For this review, take the finished solid that the model builds, in its own axes (mm). Face numbers are marked on the shaded views. A direction names the side the tool comes from. Give positions to 0.01 mm unless a question says otherwise; leave off trailing zeros. Write each loop counter-clockwise with the first axis right and the second up, starting at its lowest first coordinate (ties: lowest second). Pieces come first, ordered by that corner, then holes.
Q1. Mouldability with a two-part tool opening along Z and no side actions: class the marked faces 1, 2 and 3 as released by +Z, released by -Z, zero draft, split by the parting line, or undercut.
Q2. We need section A-A (x = 0). Write out the cut boundary in (y, z), then the cut area to 3 significant figures.
Q3. Machinability: for the marked faces 4 and 5, which of the approach directions +Z, -Z, +X, -X, +Y, -Y give a long, thin tool a straight path to every point of the face, cutting with its end or side? Answer none if there is none.
Q4. We need section B-B (z = 0). Write out the cut boundary in (x, y).
Q5. For line 1 (Y direction, x = 0.6, z = -0.15); line 2 (Y direction, x = 1.8, z = 0.45); line 3 (Z direction, x = -0.05, y = 1), list the stretches that pass through material, from the lowest coordinate up.
Q6. Insertion check: P1, Ø1, axis at x = -1, y = 8.5, coming from the +Z side; P2, Ø1, axis at y = 9, z = 1, coming from the +X side; P3, Ø1.5, axis at y = 3.5, z = 1, coming from the -X side. Each pin has a flat end and moves straight along its axis. Give the tip position at first contact, or say it passes through.
Q7. We need section C-C (y = 3). Write out the cut boundary in (x, z), then the cut area to 3 significant figures.
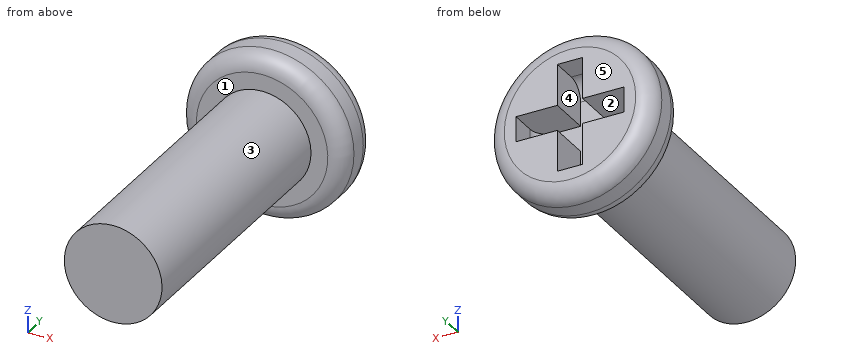
```python
from build123d import *

# Parameters (mm, degrees)
SKETCH1_R           = 1.45
BOSS_EXTRUDE1_DEPTH = 8
SKETCH2_R           = 2.45
BOSS_EXTRUDE2_DEPTH = 1.5
FILLET1_R           = 0.5
SKETCH3_W           = 0.75
SKETCH3_H           = 1.225
SKETCH3_H_2         = 0.75
SKETCH3_W_2         = 1.225
CUT_EXTRUDE1_DEPTH  = 1.25
FILLET4_R           = 0.5


with BuildPart() as part:
    # Sketch1 → Boss-Extrude1 (new body)
    with BuildSketch(Plane(origin=(0, 0, 0), x_dir=(1, 0, 0), z_dir=(0, 1, 0))):
        with Locations(Location((0, 0, 0), (0, 0, 270))):
            Circle(SKETCH1_R)
    extrude(amount=BOSS_EXTRUDE1_DEPTH)

    # Sketch2 → Boss-Extrude2 (add)
    with BuildSketch(Plane(origin=(0, 8, 0), x_dir=(1, 0, 0), z_dir=(0, 1, 0))):
        with Locations(Location((0, 0, 0), (0, 0, 270))):
            Circle(SKETCH2_R)
    extrude(amount=BOSS_EXTRUDE2_DEPTH)

    # Fillet1
    fillet1_edges = [part.edges().sort_by_distance(p)[0] for p in [
        (0, 8, -2.45),
        (0, 9.5, -2.45),
    ]]
    fillet(fillet1_edges, radius=FILLET1_R)

    # Sketch3 → Cut-Extrude1 (cut)
    with BuildSketch(Plane(origin=(0, 9.5, 0), x_dir=(1, 0, 0), z_dir=(0, 1, 0))):
        with Locations((0, 0.9875)):
            Rectangle(SKETCH3_W, SKETCH3_H)
        Rectangle(SKETCH3_W, SKETCH3_H_2)
        with Locations((0, -0.9875)):
            Rectangle(SKETCH3_W, SKETCH3_H)
        with Locations((0.9875, 0)):
            Rectangle(SKETCH3_W_2, SKETCH3_H_2)
        with Locations((-0.9875, 0)):
            Rectangle(SKETCH3_W_2, SKETCH3_H_2)
    extrude(amount=-CUT_EXTRUDE1_DEPTH, mode=Mode.SUBTRACT)

    # Fillet4
    fillet4_edges = [part.edges().sort_by_distance(p)[0] for p in [
        (0, 8.25, 1.6),
        (-1.6, 8.25, 0),
        (0, 8.25, -1.6),
        (1.6, 8.25, 0),
    ]]
    fillet(fillet4_edges, radius=FILLET4_R)


solid = part.part
```
Computed:
1. face 1: zero draft
1. face 2: undercut
1. face 3: split by the parting line
2. outline: (0, -1.45) - (8, -1.45) - (8, -1.95) arc R0.5 ccw to (8.5, -2.45) - (9, -2.45) arc R0.5 ccw to (9.5, -1.95) - (9.5, -1.6) - (8.75, -1.6) arc R0.5 cw to (8.25, -1.1) - (8.25, 1.1) arc R0.5 cw to (8.75, 1.6) - (9.5, 1.6) - (9.5, 1.95) arc R0.5 ccw to (9, 2.45) - (8.5, 2.45) arc R0.5 ccw to (8, 1.95) - (8, 1.45) - (0, 1.45) - close
2. area: 26.4 mm2
3. face 4: +Y
3. face 5: +Z, -Z, +X, -X, +Y
4. outline: (-2.45, 8.5) arc R0.5 ccw to (-1.95, 8) - (-1.45, 8) - (-1.45, 0) - (1.45, 0) - (1.45, 8) - (1.95, 8) arc R0.5 ccw to (2.45, 8.5) - (2.45, 9) arc R0.5 ccw to (1.95, 9.5) - (1.6, 9.5) - (1.6, 8.75) arc R0.5 cw to (1.1, 8.25) - (-1.1, 8.25) arc R0.5 cw to (-1.6, 8.75) - (-1.6, 9.5) - (-1.95, 9.5) arc R0.5 ccw to (-2.45, 9) - close
5. line 1: y = 0 to 8.25
5. line 2: y = 8 to 9.5
5. line 3: z = -1.45 to 1.45
6. P1: stops at z = 2.4
6. P2: stops at x = 2.4
6. P3: stops at x = -1.43
7. outline: circle Ø2.9 at (0, 0)
7. area: 6.61 mm2
